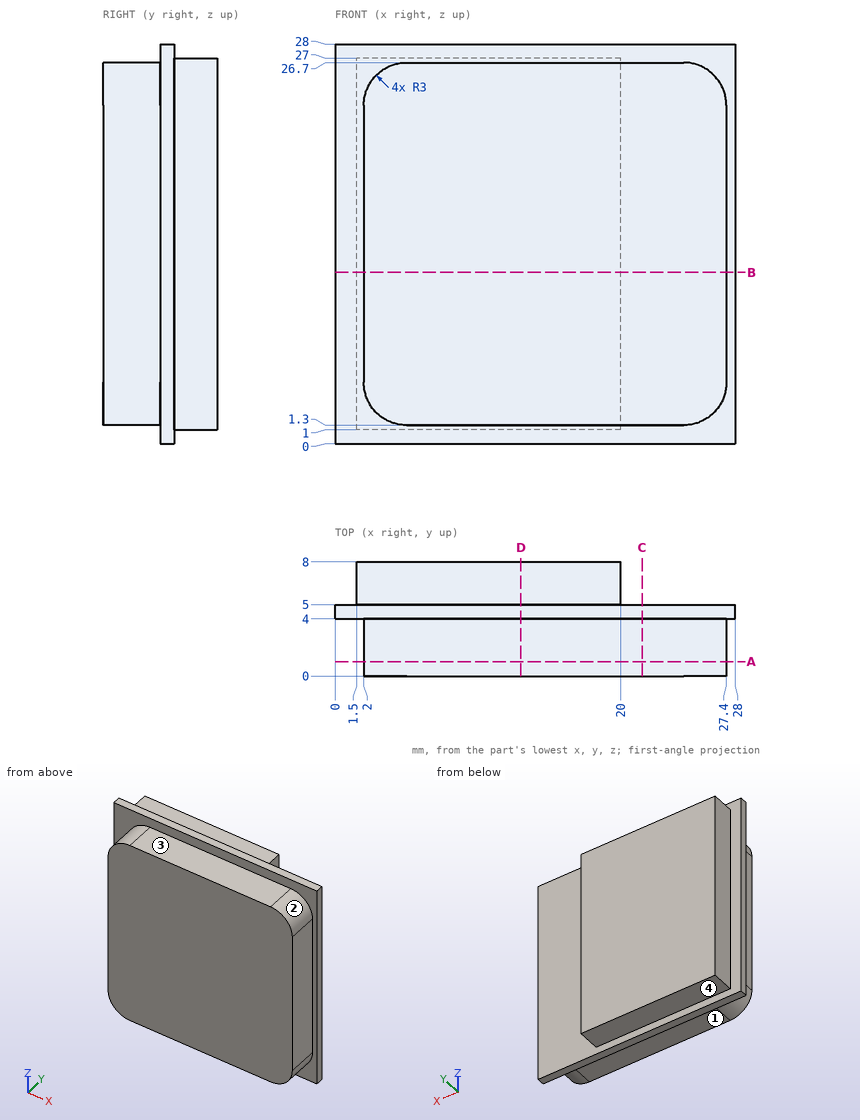
Geometry check sheet. Reference: drawing and pictorial views, mm from the part's lowest x, y, z. A direction names the side the tool comes from. Round coordinates to 2 decimals unless told otherwise and drop trailing zeros. Loops run counter-clockwise (first coordinate to the right, second up) from the corner with the lowest first, then second, coordinate; pieces in that order, holes last. Notation, with made-up numbers: (82.5, -26) -> (110.5, -26) arc R7 ccw to (110.5, -17) -> close; hole circle Ø5 at (-38.75, 17). An arc over 180 degrees is marked (long way). Answer as a JSON object with one key per item and string values.
Q1. Section check D-D (x = 13). Record the boundary of the cut face in (y, z), then the cut area to 3 significant figures.
Data:
{"outline": "(0, 1.3) -> (4, 1.3) -> (4, 0) -> (5, 0) -> (5, 1) -> (8, 1) -> (8, 27) -> (5, 27) -> (5, 28) -> (4, 28) -> (4, 26.7) -> (0, 26.7) -> close", "area": "208 mm2"}
Q2. Section check C-C (x = 21.5). Record the boundary of the cut face in (y, z), then the cut area to 3 significant figures.
Data:
{"outline": "(0, 1.3) -> (4, 1.3) -> (4, 0) -> (5, 0) -> (5, 28) -> (4, 28) -> (4, 26.7) -> (0, 26.7) -> close", "area": "130 mm2"}
Q3. Section check A-A (y = 1). Record the boundary of the cut face in (x, z), then the cut area to 3 significant figures.
Data:
{"outline": "(2, 4.3) arc R3 ccw to (5, 1.3) -> (24.4, 1.3) arc R3 ccw to (27.4, 4.3) -> (27.4, 23.7) arc R3 ccw to (24.4, 26.7) -> (5, 26.7) arc R3 ccw to (2, 23.7) -> close", "area": "637 mm2"}
Q4. Go/stop test with flat-tipped pins: P1, Ø1.5, axis at x = 4.5, y = 1.5, coming from the +Z side; P2, Ø1.2, axis at x = 11, y = 2, coming from the -Z side; P3, Ø1.2, axis at y = 2.5, z = 11, coming from the -X side. Record where each tip stops, or that it passes through.
Data:
{"P1": "stops at z = 26.7", "P2": "stops at z = 1.3", "P3": "stops at x = 2"}
Q5. Access from +Z, -Z, +X, -X, +Y, -Y to the whole of each face (thin tool, end or side, straight path). Record for the marked faces 1, 2, 3 and 4.
Data:
{"face 1": "-Z, +X, -X, -Y", "face 2": "+Z, +X, -Y", "face 3": "+Z, +X, -X, -Y", "face 4": "-Z, +X, -X, +Y"}
Q6. Scan lines: line 1 (Z direction, x = 18.25, y = 3); line 2 (X direction, y = 0.5, z = 8.75); line 3 (Z direction, x = 2, y = 5.5). Record each from-to range of solid material in increasing order. Write a range as from..to.
Data:
{"line 1": "z = 1.3..26.7", "line 2": "x = 2..27.4", "line 3": "z = 1..27"}
Q7. Section check B-B (z = 12). Record the boundary of the cut face in (x, y).
Data:
{"outline": "(0, 4) -> (2, 4) -> (2, 0) -> (27.4, 0) -> (27.4, 4) -> (28, 4) -> (28, 5) -> (20, 5) -> (20, 8) -> (1.5, 8) -> (1.5, 5) -> (0, 5) -> close"}
